from build123d import *

# Parameters (mm, degrees)
SKETCH_W        = 50
SKETCH_H        = 25
PAD_DEPTH       = 10
SKETCH001_W     = 50
SKETCH001_H     = 10.5
POCKET_DEPTH    = 2
SKETCH002_W     = 6
SKETCH002_H     = 15
POCKET001_DEPTH = 5
SKETCH003_W     = 6
SKETCH003_H     = 2.75
POCKET002_DEPTH = 5
CHAMFER_SIZE    = 0.6


with BuildPart() as part:
    # Sketch → Pad (new body)
    with BuildSketch(Plane.XY):
        with Locations((25, 12.5)):
            Rectangle(SKETCH_W, SKETCH_H)
    extrude(amount=PAD_DEPTH)

    # Sketch001 (on Face6 of Pad) → Pocket (cut)
    with BuildSketch(Plane.XY.offset(10)):
        with Locations((25, 12.5)):
            Rectangle(SKETCH001_W, SKETCH001_H)
    extrude(amount=-POCKET_DEPTH, mode=Mode.SUBTRACT)

    # Sketch002 (on Face9 of Pocket) → Pocket001 (cut)
    with BuildSketch(Plane.XY.offset(10)):
        with Locations((10.5, 12.5)):
            Rectangle(SKETCH002_W, SKETCH002_H)
        with Locations((39.5, 12.5)):
            Rectangle(SKETCH002_W, SKETCH002_H)
    extrude(amount=-POCKET001_DEPTH, mode=Mode.SUBTRACT)

    # Sketch003 (on Face24 of Pocket001) → Pocket002 (cut)
    with BuildSketch(Plane.XY.offset(5)):
        with Locations((10.5, 18.625)):
            Rectangle(SKETCH003_W, SKETCH003_H)
        with Locations((39.5, 18.625)):
            Rectangle(SKETCH003_W, SKETCH003_H)
    extrude(amount=-POCKET002_DEPTH, mode=Mode.SUBTRACT)

    # Chamfer
    chamfer_edges = [part.edges().sort_by_distance(p)[0] for p in [
        (25, 25, 10),
        (0, 21.375, 10),
        (3.75, 17.75, 10),
        (7.5, 18.875, 10),
        (10.5, 20, 10),
        (13.5, 18.875, 10),
        (25, 17.75, 10),
        (36.5, 18.875, 10),
        (39.5, 20, 10),
        (46.25, 17.75, 10),
        (50, 21.375, 10),
        (50, 12.5, 8),
        (50, 17.75, 9),
        (42.5, 12.5, 8),
        (46.25, 7.25, 10),
        (50, 7.25, 9),
        (42.5, 6.125, 10),
        (39.5, 5, 10),
        (36.5, 6.125, 10),
        (25, 7.25, 10),
        (13.5, 6.125, 10),
        (10.5, 5, 10),
        (7.5, 6.125, 10),
        (3.75, 7.25, 10),
        (7.5, 12.5, 8),
        (13.5, 12.5, 8),
        (36.5, 12.5, 8),
        (0, 12.5, 8),
        (0, 17.75, 9),
        (0, 7.25, 9),
        (0, 3.625, 10),
        (25, 0, 10),
        (50, 3.625, 10),
        (42.5, 18.875, 10),
        (7.5, 7.25, 9),
        (7.5, 17.75, 9),
        (13.5, 7.25, 9),
        (36.5, 7.25, 9),
        (36.5, 17.75, 9),
        (42.5, 17.75, 9),
        (42.5, 7.25, 9),
        (13.5, 17.75, 9),
        (0, 0, 5),
        (0, 25, 5),
        (50, 0, 5),
        (50, 25, 5),
        (39.5, 17.25, 5),
        (10.5, 17.25, 5),
    ]]
    chamfer(chamfer_edges, length=CHAMFER_SIZE)


solid = part.part
Read the model definition and answer for the solid it produces. Units are mm, in the model's axes. A direction names the side the tool comes from. Round coordinates to 2 decimals unless told otherwise and drop trailing zeros. Loops run counter-clockwise (first coordinate to the right, second up) from the corner with the lowest first, then second, coordinate; pieces in that order, holes last. Notation, with made-up numbers: (7, 54.5) - (28, 54.5) arc R21 cw to (28, 70.5) - close; hole circle Ø4 at (11, -12.75). An arc over 180 degrees is marked (long way). One line per question, with ' | ' between items. Start each with the question number.
Q1. Find the intervals of material crossed by L1, parallel to Y at x = 10, z = 5.5; L2, parallel to Y at x = 21, z = 8.5; L3, parallel to X at y = 11.5, z = 5.5, in increasing order.
Q2. Section D-D on x = 44 is taken. Give the vertices of the cut face in (y, z), plus the area to 3 significant figures.
Q3. Flat-ended cylindrical pins translate along their axes: pin 1 (6 mm diameter, centred on x = 14, y = 11.5, fed in from +Z); pin 2 (5 mm diameter, centred on x = 26.5, y = 22.5, fed in from -Z); pin 3 (1.8 mm diameter, centred on x = 9.5, y = 9.5, fed in from +Z). Find the tip coordinate at first contact, or state that the pin passes through.
Q4. Section C-C on y = 14.5 is taken. Give the vertices of the cut face in (x, z).
Q5. Section A-A on z = 3.75 is taken. Give the vertices of the cut face in (x, y), plus the area to 3 significant figures.
Q6. For a pull along Y with two mould halves and no side action, classify faces 1 (the flat face through (25, 25, 5)), 2 (the flat face through (0, 12, 5)), 3 (the flat face through (36.5, 14, 6)), 4 (the flat face through (4, 17.75, 9)) as +Y half, -Y half, draft (parallel to the pull), parting line (faces both ways), or undercut.
Q7. Section B-B on x = 8 is taken. Give the vertices of the cut face in (y, z).
Q8. For faces 5 (the flat face through (46, 7.25, 9)), 6 (the flat face through (7.5, 14, 6)), 7 (the flat face through (39, 20, 5)), determine the directions among +Z, -Z, +X, -X, +Y, -Y from which every point of the face is accessible in a straight line to the end or side of a thin tool.
Established:
1) L1: 0 to 5, 20 to 25 | L2: 0 to 7.25, 17.75 to 25 | L3: 0 to 7.5, 13.5 to 36.5, 42.5 to 50
2) outline: (0, 0) - (25, 0) - (25, 9.4) - (24.4, 10) - (18.35, 10) - (17.75, 9.4) - (17.75, 8) - (7.25, 8) - (7.25, 9.4) - (6.65, 10) - (0.6, 10) - (0, 9.4) - close | area: 228 mm²
3) pin 1: z = 8 | pin 2: z = 0 | pin 3: z = 5
4) outline: (0, 0) - (50, 0) - (50, 7.4) - (49.4, 8) - (43.1, 8) - (42.5, 7.4) - (42.5, 5) - (36.5, 5) - (36.5, 7.4) - (35.9, 8) - (14.1, 8) - (13.5, 7.4) - (13.5, 5) - (7.5, 5) - (7.5, 7.4) - (6.9, 8) - (0.6, 8) - (0, 7.4) - close
5) outline: (0, 0.6) - (0.6, 0) - (49.4, 0) - (50, 0.6) - (50, 24.4) - (49.4, 25) - (0.6, 25) - (0, 24.4) - close; hole (7.5, 17.25) - (13.5, 17.25) - (13.5, 20) - (7.5, 20) - close; hole (36.5, 17.25) - (42.5, 17.25) - (42.5, 20) - (36.5, 20) - close | area: 1,220 mm²
6) face 1: +Y half | face 2: draft | face 3: undercut | face 4: undercut
7) outline: (0, 0) - (17.25, 0) - (17.25, 4.4) - (16.65, 5) - (5, 5) - (5, 9.4) - (4.4, 10) - (0.6, 10) - (0, 9.4) - close; (20, 0) - (25, 0) - (25, 9.4) - (24.4, 10) - (20.6, 10) - (20, 9.4) - close
8) face 5: +Z, +X, -X | face 6: +Z | face 7: +Z, -Z
